from build123d import *

# Parameters (mm, degrees)
SKETCH1_W           = 40
SKETCH1_H           = 35
BOSS_EXTRUDE1_DEPTH = 3
SKETCH2_W           = 5
SKETCH2_H           = 35
BOSS_EXTRUDE2_DEPTH = 70
FILLET1_R           = 10
SKETCH3_R           = 7
CUT_EXTRUDE1_DEPTH  = 120


with BuildPart() as part:
    # Sketch1 → Boss-Extrude1 (new body)
    with BuildSketch(Plane(origin=(0, 0, 0), x_dir=(0, 0, -1), z_dir=(1, 0, 0))):
        with Locations((-20, 17.5)):
            Rectangle(SKETCH1_W, SKETCH1_H)
    extrude(amount=BOSS_EXTRUDE1_DEPTH)

    # Sketch2 → Boss-Extrude2 (add)
    with BuildSketch(Plane(origin=(0, 0, 0), x_dir=(0, 0, -1), z_dir=(1, 0, 0))):
        with Locations((-37.5, 17.5)):
            Rectangle(SKETCH2_W, SKETCH2_H)
        with Locations((-2.5, 17.5)):
            Rectangle(SKETCH2_W, SKETCH2_H)
    extrude(amount=BOSS_EXTRUDE2_DEPTH)

    # Fillet1
    fillet1_edges = [part.edges().sort_by_distance(p)[0] for p in [
        (70, 35, 37.5),
        (70, 0, 37.5),
        (70, 0, 2.5),
        (70, 35, 2.5),
    ]]
    fillet(fillet1_edges, radius=FILLET1_R)

    # Sketch3 → Cut-Extrude1 (cut)
    with BuildSketch(Plane.XY.offset(40)):
        with Locations(Location((55, 17.5, 0), (0, 0, 90))):
            Circle(SKETCH3_R)
    extrude(amount=-CUT_EXTRUDE1_DEPTH, mode=Mode.SUBTRACT)


solid = part.part
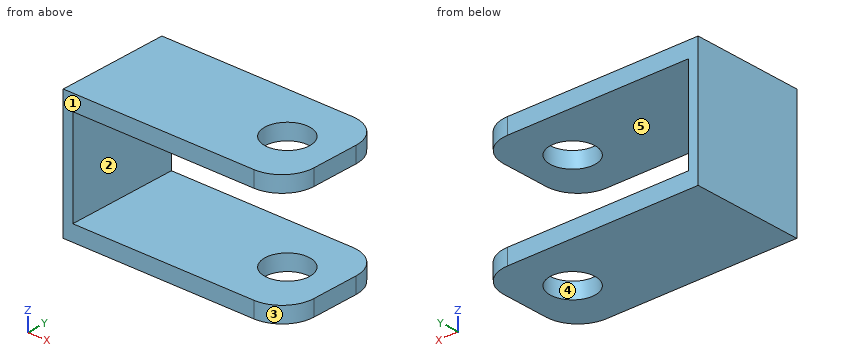
Source: CAD feature listing. Evaluate the final solid. Frame: model axes, mm. Face numbers are marked on the shaded views. A direction names the side the tool comes from. Coordinates: 2 decimals unless noted, no trailing zeros. Loops run counter-clockwise (first coordinate to the right, second up) from the corner with the lowest first, then second, coordinate; pieces in that order, holes last. Notation, with made-up numbers: M -5,15.25 L 47,15.25 A17 ccw 47,31.25 Z; hole C 19,42 d5. An arc over 180 degrees is marked long. Answer in a Markdown table with one row per item.
Q1. First-contact query: pin 1 (1 mm diameter, centred on y = 5, z = 7.5, fed in from +X); pin 2 (12.5 mm diameter, centred on x = 55, y = 17.5, fed in from +Z). Flat tips, straight axial feed; report the tip coordinate or a pass-through.
Answers below:
| item | result |
|---|---|
| pin 1 | stops at x = 3 |
| pin 2 | passes through |
Q2. Section B-B on y = 17.5. Return the cut outline in (x, z), plus the area to 3 significant figures.
Answers below:
| item | result |
|---|---|
| outline | M 0,0 L 48,0 L 48,5 L 3,5 L 3,35 L 48,35 L 48,40 L 0,40 Z; M 62,0 L 70,0 L 70,5 L 62,5 Z; M 62,35 L 70,35 L 70,40 L 62,40 Z |
| area | 650 mm^2 |
Q3. Set-up query: the marked faces 1 and 2. Return all of +Z, -Z, +X, -X, +Y, -Y with unobstructed straight access to the full face (end or side cutting, diameter ignored); none if empty.
Answers below:
| item | result |
|---|---|
| face 1 | +Z, -Z, +X, -X, -Y |
| face 2 | +X, +Y, -Y |
Q4. Ray query, probe 1 along Z at (x, y) = (23.5, 10); probe 2 along X at (y, z) = (17.5, 36.9); probe 3 along Y at (x, z) = (55, 2). Return the intervals inside material, ascending. Write a range as from..to.
Answers below:
| item | result |
|---|---|
| probe 1 | z = 0..5, 35..40 |
| probe 2 | x = 0..48, 62..70 |
| probe 3 | y = 0..10.5, 24.5..35 |
Q5. Section A-A on x = 55. Return the cut outline in (y, z).
Answers below:
| item | result |
|---|---|
| outline | M 0,0 L 10.5,0 L 10.5,5 L 0,5 Z; M 0,35 L 10.5,35 L 10.5,40 L 0,40 Z; M 24.5,0 L 35,0 L 35,5 L 24.5,5 Z; M 24.5,35 L 35,35 L 35,40 L 24.5,40 Z |
Q6. Section D-D on z = 36. Return the cut outline in (x, y), plus the area to 3 significant figures.
Answers below:
| item | result |
|---|---|
| outline | M 0,0 L 60,0 A10 ccw 70,10 L 70,25 A10 ccw 60,35 L 0,35 Z; hole C 55,17.5 d14 |
| area | 2,250 mm^2 |
Q7. Draft query along X for the marked faces 3, 4 and 5. Return one class per face: pulls with the +X half, pulls with the -X half, needs draft (parallel to the pull), parting line crosses it, or undercut.
Answers below:
| item | result |
|---|---|
| face 3 | pulls with the +X half |
| face 4 | undercut |
| face 5 | needs draft |
Q8. Section C-C on x = 18.5. Return the cut outline in (y, z).
Answers below:
| item | result |
|---|---|
| outline | M 0,0 L 35,0 L 35,5 L 0,5 Z; M 0,35 L 35,35 L 35,40 L 0,40 Z |
